from build123d import *

# Parameters (mm, degrees)
RESSALTO_EXTRUS_O1_DEPTH = 15
ESBO_O3_R                = 1.1
CORTE_EXTRUS_O1_DEPTH    = 30
CORTE_EXTRUS_O8_DEPTH    = 1
ESBO_O16_R               = 1.1
CORTE_EXTRUS_O9_DEPTH    = 7
ESBO_O17_R               = 1.6
CORTE_EXTRUS_O10_DEPTH   = 3
ESBO_O18_R               = 1.6
CORTE_EXTRUS_O11_DEPTH   = 15
ESBO_O19_R               = 2.075
CORTE_EXTRUS_O12_DEPTH   = 4
ESBO_O20_R               = 2.2
CORTE_EXTRUS_O13_DEPTH   = 2


with BuildPart() as part:
    # Esboço1 → Ressalto-extrusão1 (new body, symmetric)
    with BuildSketch(Plane(origin=(0, 0, 0), x_dir=(0, 0, -1), z_dir=(1, 0, 0))):
        Polygon((0, 0), (0, -18), (-18, -18), (-18, -24), (7, -24), (7, 0), align=None)
    extrude(amount=RESSALTO_EXTRUS_O1_DEPTH, both=True)

    # Esboço3 → Corte-extrusão1 (cut)
    with BuildSketch(Plane.XZ.offset(18)):
        with Locations((-6.5, 15.5)):
            Circle(ESBO_O3_R)
        with Locations((6.5, 15.5)):
            Circle(ESBO_O3_R)
        with Locations((6.5, 3.5)):
            Circle(ESBO_O3_R)
        with Locations((-6.5, 3.5)):
            Circle(ESBO_O3_R)
    extrude(amount=CORTE_EXTRUS_O1_DEPTH, mode=Mode.SUBTRACT)

    # Esboço15 → Corte-extrusão8 (cut)
    with BuildSketch(Plane.XY):
        with BuildLine():
            Line((-1.870828693, -4.5), (-15, -4.5))
            Line((-15, -4.5), (-15, -5.5))
            Line((-15, -5.5), (-1.870828693, -5.5))
            ThreePointArc((-1.870828693, -5.5), (0, -9), (1.870828693, -5.5))
            Line((1.870828693, -5.5), (15, -5.5))
            Line((15, -5.5), (15, -4.5))
            Line((15, -4.5), (1.870828693, -4.5))
            Line((1.870828693, -4.5), (-1.870828693, -4.5))
        make_face()
        with BuildLine():
            Line((15, -0.5), (1.870828693, -0.5))
            ThreePointArc((1.870828693, -0.5), (0, -4), (-1.870828693, -0.5))
            Line((-1.870828693, -0.5), (-15, -0.5))
            Line((-15, -0.5), (-15, 0.5))
            Line((-15, 0.5), (-1.870828693, 0.5))
            Line((-1.870828693, 0.5), (1.870828693, 0.5))
            Line((1.870828693, 0.5), (15, 0.5))
            Line((15, 0.5), (15, -0.5))
        make_face()
    extrude(amount=-CORTE_EXTRUS_O8_DEPTH, mode=Mode.SUBTRACT)

    # Esboço16 → Corte-extrusão9 (cut)
    with BuildSketch(Plane.XY):
        with Locations((0, -1.75)):
            Circle(ESBO_O16_R)
        with Locations((0, -6.75)):
            Circle(ESBO_O16_R)
    extrude(amount=-CORTE_EXTRUS_O9_DEPTH, mode=Mode.SUBTRACT)

    # Esboço17 → Corte-extrusão10 (cut)
    with BuildSketch(Plane(origin=(0, 0, -7), x_dir=(-1, 0, 0), z_dir=(0, 0, -1))):
        with Locations((0, -1.75)):
            Circle(ESBO_O17_R)
        with Locations((0, -6.75)):
            Circle(ESBO_O17_R)
    extrude(amount=-CORTE_EXTRUS_O10_DEPTH, mode=Mode.SUBTRACT)

    # Esboço18 → Corte-extrusão11 (cut)
    with BuildSketch(Plane(origin=(0, 0, -7), x_dir=(-1, 0, 0), z_dir=(0, 0, -1))):
        with Locations((12.5, -21)):
            Circle(ESBO_O18_R)
        with Locations((-12.5, -21)):
            Circle(ESBO_O18_R)
    extrude(amount=-CORTE_EXTRUS_O11_DEPTH, mode=Mode.SUBTRACT)

    # Esboço19 → Corte-extrusão12 (cut)
    with BuildSketch(Plane(origin=(0, 0, -7), x_dir=(-1, 0, 0), z_dir=(0, 0, -1))):
        with Locations((12.5, -21)):
            Circle(ESBO_O19_R)
        with Locations((-12.5, -21)):
            Circle(ESBO_O19_R)
    extrude(amount=-CORTE_EXTRUS_O12_DEPTH, mode=Mode.SUBTRACT)

    # Esboço20 → Corte-extrusão13 (cut)
    with BuildSketch(Plane.XZ.offset(24)):
        with Locations((-6.5, 15.5)):
            Circle(ESBO_O20_R)
        with Locations((6.5, 15.5)):
            Circle(ESBO_O20_R)
        with Locations((6.5, 3.5)):
            Circle(ESBO_O20_R)
        with Locations((-6.5, 3.5)):
            Circle(ESBO_O20_R)
    extrude(amount=-CORTE_EXTRUS_O13_DEPTH, mode=Mode.SUBTRACT)


solid = part.part
Can you work these out from the model? Positions are in its coordinate system, mm. A direction names the side the tool comes from. Coordinates: 2 decimals unless noted, no trailing zeros. Write each loop counter-clockwise with the first axis right and the second up, starting at its lowest first coordinate (ties: lowest second). Pieces come first, ordered by that corner, then holes.
Q1. Which directions (+Z, -Z, +X, -X, +Y, -Y) give clear straight access to the entire face, cutting with the end or side of a thin tool? Please do faces 3 (the face through (13, -21, 8)), 4 (the face through (7, -22, 5)), 5 (the face through (-0.07, -9, -0.49)).
Results found:
face 3: -Z
face 4: -Y
face 5: +Z
Q2. For P1, Ø2.5, axis at x = 6.5, z = 3.5, coming from the +Y side; P2, Ø1, axis at x = 0, y = -11, coming from the +Z side; P3, Ø4, axis at x = -6.5, z = 15.5, coming from the -Y side; P4, Ø2, axis at x = -6.5, z = 3.5, coming from the +Y side, each with a flat end and sliding along its axis, tell me the tip position at first contact or that it passes through.
Results found:
P1: stops at y = -18
P2: stops at z = 0
P3: stops at y = -22
P4: passes through
Q3. Imagine slicing it at C-C, the plane y = -1.75. List the corners of the cut face in (x, z) for me, plus the area to 3 significant figures.
Results found:
outline: (-15, -7) - (-1.6, -7) - (-1.6, -4) - (-1.1, -4) - (-1.1, -1) - (-2.25, -1) - (-2.25, 0) - (-15, 0) - close; (1.1, -4) - (1.6, -4) - (1.6, -7) - (15, -7) - (15, 0) - (2.25, 0) - (2.25, -1) - (1.1, -1) - close
area: 189 mm2
Q4. Please list where these lines run through material, in increasing order: L1, parallel to Z at x = -6.5, y = -22.5; L2, parallel to X at y = -19.35, z = 3.5; L3, parallel to X at y = -1.75, z = -0.4.
Results found:
L1: z = -7 to 1.3, 5.7 to 13.3, 17.7 to 18
L2: x = -15 to -7.6, -5.4 to 5.4, 7.6 to 15
L3: x = -15 to -2.25, 2.25 to 15
Q5. Imagine slicing it at A-A, the plane x = 6.5. List the corners of the cut face in (y, z) for me.
Results found:
outline: (-24, -7) - (0, -7) - (0, -1) - (-0.5, -1) - (-0.5, 0) - (-4.5, 0) - (-4.5, -1) - (-5.5, -1) - (-5.5, 0) - (-18, 0) - (-18, 2.4) - (-22, 2.4) - (-22, 1.3) - (-24, 1.3) - close; (-24, 5.7) - (-22, 5.7) - (-22, 4.6) - (-18, 4.6) - (-18, 14.4) - (-22, 14.4) - (-22, 13.3) - (-24, 13.3) - close; (-24, 17.7) - (-22, 17.7) - (-22, 16.6) - (-18, 16.6) - (-18, 18) - (-24, 18) - close
Q6. If we mould it in two halves opening along X, with no side actions, what happens to faces 1 (the face through (0, -5, -1)), 2 (the face through (0.2, -4.5, -0.5))? For each: +X half, -X half, draft (parallel to the pull), parting line (faces both ways), or undercut.
Results found:
face 1: undercut
face 2: draft
Q7. Imagine slicing it at D-D, the plane x = 12.5. List the corners of the cut face in (y, z) for me (3 decimals), plus the area to 3 significant figures.
Results found:
outline: (-24, -7) - (-23.075, -7) - (-23.075, -3) - (-22.6, -3) - (-22.6, 8) - (-19.4, 8) - (-19.4, -3) - (-18.925, -3) - (-18.925, -7) - (0, -7) - (0, -1) - (-0.5, -1) - (-0.5, 0) - (-4.5, 0) - (-4.5, -1) - (-5.5, -1) - (-5.5, 0) - (-18, 0) - (-18, 18) - (-24, 18) - close
area: 223 mm2
Q8. Imagine slicing it at B-B, the plane z = 15.5. List the corners of the cut face in (x, y) for me, plus the area to 3 significant figures.
Results found:
outline: (-15, -24) - (-8.7, -24) - (-8.7, -22) - (-7.6, -22) - (-7.6, -18) - (-15, -18) - close; (-5.4, -22) - (-4.3, -22) - (-4.3, -24) - (4.3, -24) - (4.3, -22) - (5.4, -22) - (5.4, -18) - (-5.4, -18) - close; (7.6, -22) - (8.7, -22) - (8.7, -24) - (15, -24) - (15, -18) - (7.6, -18) - close
area: 145 mm2
